```python
from build123d import *

# Parameters (mm, degrees)
F1_DEPTH  = 10
F2_R      = 10
F3_DEPTH  = 25
F4_W      = 50
F4_H      = 10
F5_DEPTH  = 580
F7_R      = 10
F8_DEPTH  = 40
F12_W     = 50
F12_H     = 50
F12_R     = 10
F13_DEPTH = 10
F14_W     = 50
F14_H     = 10
F14_W_2   = 71.0721209645
F15_DEPTH = 10
F16_DEPTH = 50


with BuildPart() as f1:
    # F0 (on Front) → F1 (new body)
    with BuildSketch(Plane.XZ):
        with BuildLine():
            Line((0, 40), (0, 0))
            Line((0, 0), (50, 0))
            Line((50, 0), (50, 40))
            ThreePointArc((50, 40), (25, 65), (0, 40))
        make_face()
    extrude(amount=F1_DEPTH)

    # F2 (on face) → F3 (cut)
    with BuildSketch(Plane(origin=(0, 0, 0), x_dir=(-1, 0, 0), z_dir=(0, 1, 0))):
        with Locations((-25, 40)):
            Circle(F2_R)
    extrude(amount=-F3_DEPTH, mode=Mode.SUBTRACT)


with BuildPart() as f5:
    # F4 (on face) → F5 (new body)
    with BuildSketch(Plane(origin=(0, 0, 0), x_dir=(-1, 0, 0), z_dir=(0, 1, 0))):
        with Locations((-25, 5)):
            Rectangle(F4_W, F4_H)
    extrude(amount=F5_DEPTH)


with BuildPart() as f6_1:
    # F6: copy of F1
    add(f1.part.moved(Location((0, 590, 0))))


with BuildPart() as f8:
    # F7 (on face) → F8 (new body)
    with BuildSketch(Plane.XZ.offset(10)):
        with Locations((25, 0)):
            Circle(F7_R)
    extrude(amount=-F8_DEPTH)


with BuildPart() as f9_1:
    # F9: copy of F8
    add(f8.part.moved(Location((0, 560, 0))))


with BuildPart() as f1_1:
    add(f1.part)

    add(f5.part)  # F13 merges F5

    add(f6_1.part)  # F13 merges F6_1
    # F12 (on face) → F13 (join)
    with BuildSketch(Plane.XY.offset(10)):
        with Locations((-25, 25)):
            Rectangle(F12_W, F12_H)
        with Locations((-25, 25)):
            Circle(F12_R, mode=Mode.SUBTRACT)
        with Locations((-25, 555)):
            Rectangle(F12_W, F12_H)
        with Locations((-25, 555)):
            Circle(F12_R, mode=Mode.SUBTRACT)
        with Locations((75, 25)):
            Rectangle(F12_W, F12_H)
        with Locations((75, 25)):
            Circle(F12_R, mode=Mode.SUBTRACT)
        with Locations((75, 555)):
            Rectangle(F12_W, F12_H)
        with Locations((75, 555)):
            Circle(F12_R, mode=Mode.SUBTRACT)
    extrude(amount=-F13_DEPTH)

    # F14 (on face) → F15 (join)
    with BuildSketch(Plane.XZ):
        with Locations((-25, 5)):
            Rectangle(F14_W, F14_H)
        with Locations((-85.5360604823, 5)):
            Rectangle(F14_W_2, F14_H)
        with BuildLine():
            Line((-121.0721209645, 10), (-50, 10))
            Line((-50, 10), (0, 10))
            Line((0, 10), (0, 90.9955129027))
            ThreePointArc((0, 90.9955129027), (-60.5360604823, 30.4594524205), (-121.0721209645, 90.9955129027))
            Line((-121.0721209645, 90.9955129027), (-121.0721209645, 10))
        make_face()
        with BuildLine():
            ThreePointArc((0, 90.9955129027), (-60.5360604823, 151.531573385), (-121.0721209645, 90.9955129027))
            Line((-121.0721209645, 90.9955129027), (-70.5360604823, 90.9955129027))
            ThreePointArc((-70.5360604823, 90.9955129027), (-60.5360604823, 100.9955129027), (-50.5360604823, 90.9955129027))
            Line((-50.5360604823, 90.9955129027), (0, 90.9955129027))
        make_face()
        with BuildLine():
            Line((-70.5360604823, 90.9955129027), (-121.0721209645, 90.9955129027))
            ThreePointArc((-121.0721209645, 90.9955129027), (-60.5360604823, 30.4594524205), (0, 90.9955129027))
            Line((0, 90.9955129027), (-50.5360604823, 90.9955129027))
            ThreePointArc((-50.5360604823, 90.9955129027), (-60.5360604823, 80.9955129027), (-70.5360604823, 90.9955129027))
        make_face()
    extrude(amount=F15_DEPTH)

    # F14 (on face) → F16 (join)
    with BuildSketch(Plane.XZ):
        with Locations((-85.5360604823, 5)):
            Rectangle(F14_W_2, F14_H)
    extrude(amount=-F16_DEPTH)


solid = f1_1.part
```
Geometry check sheet. Reference: the model listing, model coordinates, mm. A direction names the side the tool comes from. Give positions to 0.01 mm unless a question says otherwise; leave off trailing zeros. Order: outer loops, then holes, each group sorted by start corner. A loop starts at its lowest first (then second) coordinate and runs counter-clockwise, first axis right, second up.
1. Access from +Z, -Z, +X, -X, +Y, -Y to the whole of each face (thin tool, end or side, straight path). Record for faces 5 (the face through (25, 580, 26)), 6 (the face through (50, 585, 20)), 7 (the face through (75, 50, 5)), 8 (the face through (-61, 50, 5)).
2. Gauge pin test, flat ends, axial feed: pin 1 Ø8 at (x, z) = (87, 6.5) entering from -Y; pin 2 Ø18 at (x, z) = (25, 40) entering from +Y; pin 3 Ø11 at (x, z) = (-53.5, 4) entering from +Y; pin 4 Ø3 at (y, z) = (582.5, 11.5) entering from -X. Record the tip position at first contact, or that the pin passes through.
3. Section check C-C, the plane x = 28. Enter the section's corners in (y, z).
4. Section check A-A, the plane y = 25. Enter the section's corners in (x, z).
5. Thickness scan on L1, parallel to X at y = 555, z = 4; L2, parallel to Y at x = 5, z = 44.5; L3, parallel to Z at x = 25, y = 586.25. Record the ranges inside material, lowest first.
6. Section check B-B, the plane x = 75. Enter the section's corners in (y, z), and give its area (3 significant figures).
7. Section check D-D, the plane y = 555. Enter the section's corners in (x, z), and give its area (3 significant figures).
8. Release check for a two-part mould opening along Y. For faces 1 (the face through (-15.46, 28, 5.07)), 2 (the face through (-25, 530, 5)), 3 (the face through (100, 555, 5)), 4 (the face through (-56, -10, 60)) record: pulls with the +Y half, pulls with the -Y half, needs draft (parallel to the pull), parting line crosses it, or undercut.
Values follow:
1. face 5: +Z, +X, -X
1. face 6: +Z, -Z, +X, +Y
1. face 7: +Z, -Z, +X
1. face 8: +Z, -Z, -X
2. pin 1: stops at y = 0
2. pin 2: passes through
2. pin 3: stops at y = 580
2. pin 4: stops at x = 0
3. outline: (-10, 0) - (590, 0) - (590, 30.46) - (580, 30.46) - (580, 10) - (0, 10) - (0, 30.46) - (-10, 30.46) - close; (-10, 49.54) - (0, 49.54) - (0, 64.82) - (-10, 64.82) - close; (580, 49.54) - (590, 49.54) - (590, 64.82) - (580, 64.82) - close
4. outline: (-121.07, 0) - (-35, 0) - (-35, 10) - (-121.07, 10) - close; (-15, 0) - (65, 0) - (65, 10) - (-15, 10) - close; (85, 0) - (100, 0) - (100, 10) - (85, 10) - close
5. L1: x = -50 to -35, -15 to 65, 85 to 100
5. L2: y = -10 to 0, 580 to 590
5. L3: z = 0 to 30, 50 to 65
6. outline: (0, 0) - (15, 0) - (15, 10) - (0, 10) - close; (35, 0) - (50, 0) - (50, 10) - (35, 10) - close; (530, 0) - (545, 0) - (545, 10) - (530, 10) - close; (565, 0) - (580, 0) - (580, 10) - (565, 10) - close
6. area: 600 mm2
7. outline: (-50, 0) - (-35, 0) - (-35, 10) - (-50, 10) - close; (-15, 0) - (65, 0) - (65, 10) - (-15, 10) - close; (85, 0) - (100, 0) - (100, 10) - (85, 10) - close
7. area: 1,100 mm2
8. face 1: undercut
8. face 2: undercut
8. face 3: needs draft
8. face 4: pulls with the -Y half
